Geometry: final body of the model. Coordinates: model frame, mm. Face numbers are marked on the shaded views. Round coordinates to 2 decimals unless told otherwise and drop trailing zeros. Write each loop counter-clockwise with the first axis right and the second up, starting at its lowest first coordinate (ties: lowest second). Pieces come first, ordered by that corner, then holes. Notation, with made-up numbers: (19.5, -22) - (51.5, -22) arc R33 cw to (51.5, 11) - close; hole circle Ø1 at (43, -29). An arc over 180 degrees is marked (long way). Use a Markdown table: item, result. Add a question column.
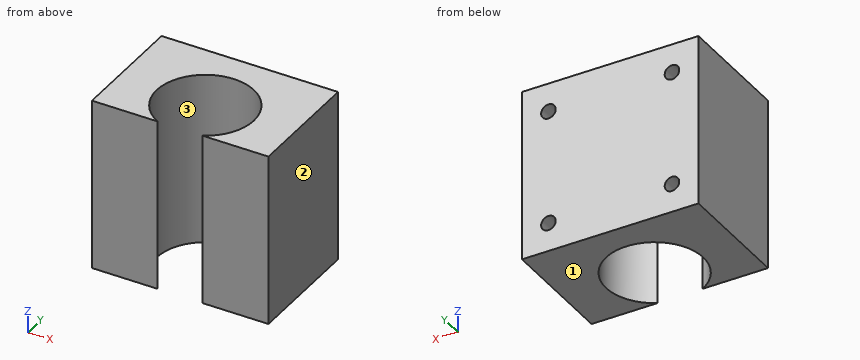
```python
from build123d import *

# Parameters (mm, degrees)
BOSS_EXTRUDE1_DEPTH = 39
SKETCH2_R           = 1.65
CUT_EXTRUDE1_DEPTH  = 5


with BuildPart() as part:
    # Sketch1 → Boss-Extrude1 (new body)
    with BuildSketch(Plane.XY):
        with BuildLine():
            Line((-20, 17.25), (20, 17.25))
            Line((20, 17.25), (20, -9.75))
            Line((20, -9.75), (5.092887197, -9.75))
            ThreePointArc((5.092887197, -9.75), (0, 11), (-5.092887197, -9.75))
            Line((-5.092887197, -9.75), (-20, -9.75))
            Line((-20, -9.75), (-20, 17.25))
        make_face()
    extrude(amount=BOSS_EXTRUDE1_DEPTH)

    # Sketch2 → Cut-Extrude1 (cut)
    with BuildSketch(Plane(origin=(0, 17.25, 0), x_dir=(1, 0, 0), z_dir=(0, 1, 0))):
        with Locations((-14, -6.5)):
            Circle(SKETCH2_R)
        with Locations((14, -6.5)):
            Circle(SKETCH2_R)
        with Locations((-14, -32.5)):
            Circle(SKETCH2_R)
        with Locations((14, -32.5)):
            Circle(SKETCH2_R)
    extrude(amount=-CUT_EXTRUDE1_DEPTH, mode=Mode.SUBTRACT)


solid = part.part
```
1) Draft query along X for the marked faces 1, 2 and 3. Return one class per face: released by +X, released by -X, zero draft, split by the parting line, or undercut.
2) Section B-B, the plane y = 15.75. Return the cut outline in (x, z).
3) Pin query (flat end, axial travel): P1, Ø1.6, axis at x = 14.5, z = 32.5, coming from the +Y side. Return the tip coordinate at first contact, or that it passes through.
4) Section A-A, the plane y = 0. Return the cut outline in (x, z).
5) Section D-D, the plane x = -6. Return the cut outline in (y, z).
6) Section C-C, the plane z = 18.5. Return the cut outline in (x, y), then the cut area to 3 significant figures.
7) Material intervals for L1, parallel to X at y = 16.15, z = 32.5; L2, parallel to Z at x = -14, y = 15.95; L3, parallel to X at y = 9.75, z = 26, sorted ascending. Write a range as from..to.
Output values:
| question | item | result |
|---|---|---|
| 1 | face 1 | zero draft |
| 1 | face 2 | released by +X |
| 1 | face 3 | undercut |
| 2 | outline | (-20, 0) - (20, 0) - (20, 39) - (-20, 39) - close; hole circle Ø3.3 at (-14, 6.5); hole circle Ø3.3 at (-14, 32.5); hole circle Ø3.3 at (14, 6.5); hole circle Ø3.3 at (14, 32.5) |
| 3 | P1 | stops at y = 12.25 |
| 4 | outline | (-20, 0) - (-11, 0) - (-11, 39) - (-20, 39) - close; (11, 0) - (20, 0) - (20, 39) - (11, 39) - close |
| 5 | outline | (-9.75, 0) - (-9.22, 0) - (-9.22, 39) - (-9.75, 39) - close; (9.22, 0) - (17.25, 0) - (17.25, 39) - (9.22, 39) - close |
| 6 | outline | (-20, -9.75) - (-5.09, -9.75) arc R11 cw (long way) to (5.09, -9.75) - (20, -9.75) - (20, 17.25) - (-20, 17.25) - close |
| 6 | area | 708 mm^2 |
| 7 | L1 | x = -20..-15.65, -12.35..12.35, 15.65..20 |
| 7 | L2 | z = 0..4.85, 8.15..30.85, 34.15..39 |
| 7 | L3 | x = -20..-5.09, 5.09..20 |
